from build123d import *

# Parameters (mm, degrees)
BOSS_EXTRUDE1_DEPTH = 165.1
SKETCH3_R           = 2.667
CUT_EXTRUDE1_DEPTH  = 165.1


with BuildPart() as part:
    # Sketch1 → Boss-Extrude1 (new body)
    with BuildSketch(Plane.XY):
        with BuildLine():
            Line((-5.08, 0), (5.08, 0))
            Line((5.08, 0), (5.08, 1.27))
            ThreePointArc((5.08, 1.27), (25.4, 15.895452724), (45.72, 1.27))
            Line((45.72, 1.27), (45.72, 0))
            Line((45.72, 0), (55.88, 0))
            Line((55.88, 0), (55.88, 3.161651537))
            Line((55.88, 3.161651537), (45.736301675, 3.161651537))
            ThreePointArc((45.736301675, 3.161651537), (25.4, 20.58060267), (5.063698325, 3.161651537))
            Line((5.063698325, 3.161651537), (-5.08, 3.161651537))
            Line((-5.08, 3.161651537), (-5.08, 0))
        make_face()
    extrude(amount=BOSS_EXTRUDE1_DEPTH)

    # Sketch3 → Cut-Extrude1 (cut)
    with BuildSketch(Plane(origin=(0, 3.161651537, 0), x_dir=(1, 0, 0), z_dir=(0, 1, 0))):
        with Locations(Location((0, -6.6675, 0), (0, 0, 270))):
            Circle(SKETCH3_R)
        with Locations(Location((0, -32.0675, 0), (0, 0, 270))):
            Circle(SKETCH3_R)
        with Locations(Location((0, -57.4675, 0), (0, 0, 270))):
            Circle(SKETCH3_R)
        with Locations(Location((0, -82.8675, 0), (0, 0, 270))):
            Circle(SKETCH3_R)
        with Locations(Location((0, -108.2675, 0), (0, 0, 270))):
            Circle(SKETCH3_R)
        with Locations(Location((0, -133.6675, 0), (0, 0, 270))):
            Circle(SKETCH3_R)
        with Locations(Location((0, -159.0675, 0), (0, 0, 270))):
            Circle(SKETCH3_R)
        with Locations(Location((50.8, -159.0675, 0), (0, 0, 180))):
            Circle(SKETCH3_R)
        with Locations(Location((50.8, -133.6675, 0), (0, 0, 180))):
            Circle(SKETCH3_R)
        with Locations(Location((50.8, -108.2675, 0), (0, 0, 180))):
            Circle(SKETCH3_R)
        with Locations(Location((50.8, -82.8675, 0), (0, 0, 180))):
            Circle(SKETCH3_R)
        with Locations(Location((50.8, -57.4675, 0), (0, 0, 180))):
            Circle(SKETCH3_R)
        with Locations(Location((50.8, -32.0675, 0), (0, 0, 180))):
            Circle(SKETCH3_R)
        with Locations(Location((50.8, -6.6675, 0), (0, 0, 180))):
            Circle(SKETCH3_R)
    extrude(amount=-CUT_EXTRUDE1_DEPTH, mode=Mode.SUBTRACT)


solid = part.part
Verification items for the finished model (mm, model axes). A direction names the side the tool comes from. Coordinates: 2 decimals unless noted, no trailing zeros. Loops run counter-clockwise (first coordinate to the right, second up) from the corner with the lowest first, then second, coordinate; pieces in that order, holes last. Notation, with made-up numbers: (29, -23.5) -> (79, -23.5) arc R28 cw to (79, -1.5) -> close; hole circle Ø1 at (83, 82). An arc over 180 degrees is marked (long way). Answer as a JSON object with one key per item and string values. Group by question number.
Item 1: Depth check by flat-ended pin: pin 1 (8.5 mm diameter, centred on x = 50.8, z = 82.87, fed in from -Y); pin 2 (1 mm diameter, centred on x = 36.5, z = 50.5, fed in from -Y); pin 3 (10 mm diameter, centred on x = 4.5, z = 33.5, fed in from +Y); pin 4 (6 mm diameter, centred on x = 0, z = 159.07, fed in from +Y). Enter the tip coordinate at first touch or a pass-through.
Item 2: Mould release check, pull along Z, two halves, no side actions. Record for faces 1 (the cylindrical face through (25.808, 20.577, 81.394)), 2 (the cylindrical face through (-1.02, 1.6, 59.93)), 3 (the flat face through (25.3, 16.4, 0)): +Z half, -Z half, draft (parallel to the pull), parting line (faces both ways), or undercut.
Item 3: Sectioned sample at B-B on y = 13.5. Record the boundary of the cut face in (x, z).
Item 4: Scan lines: probe 1 along X at (y, z) = (12.5, 99); probe 2 along Y at (x, z) = (49, 146); probe 3 along X at (y, z) = (5.75, 69). Record each from-to range of solid material in increasing order.
Item 5: Sectioned sample at C-C on z = 99. Record the boundary of the cut face in (x, y), plus the area to 3 significant figures.
Item 6: Tool access check on faces 4 (the cylindrical face through (-1.02, 1.6, 34.53)), 5 (the flat face through (3, 3.162, 81)), 6 (the flat face through (53, 3.162, 81)). Record the directions out of +Z, -Z, +X, -X, +Y, -Y that give a thin tool (end or side, any length) a straight path to the whole face; none if there is none.
Item 7: Sectioned sample at A-A on x = 50.8. State how many separate pieces and enclosed holes the cut face has, plus the area to 3 significant figures.
Item 8: Sectioned sample at D-D on x = 44. Record the boundary of the cut face in (y, z).
Evaluation:
{
 "1": {"pin 1": "stops at y = 0", "pin 2": "stops at y = 12.48", "pin 3": "stops at y = 13.07", "pin 4": "stops at y = 3.16"},
 "2": {"face 1": "draft", "face 2": "undercut", "face 3": "-Z half"},
 "3": {"outline": "(9.87, 0) -> (15.55, 0) -> (15.55, 165.1) -> (9.87, 165.1) -> close; (35.25, 0) -> (40.93, 0) -> (40.93, 165.1) -> (35.25, 165.1) -> close"},
 "4": {"probe 1": "x = 9.05 to 13.82, 36.98 to 41.75", "probe 2": "y = 0 to 3.16", "probe 3": "x = 5.64 to 7.18, 43.62 to 45.16"},
 "5": {"outline": "(-5.08, 0) -> (5.08, 0) -> (5.08, 1.27) arc R21.43 cw to (45.72, 1.27) -> (45.72, 0) -> (55.88, 0) -> (55.88, 3.16) -> (45.74, 3.16) arc R20.58 ccw to (5.06, 3.16) -> (-5.08, 3.16) -> close", "area": "242 mm²"},
 "6": {"face 4": "+Y, -Y", "face 5": "+Z, -Z, -X, +Y", "face 6": "+Z, -Z, +X, +Y"},
 "7": {"separate pieces": "8", "enclosed holes": "0", "area": "404 mm²"},
 "8": {"outline": "(5.11, 0) -> (8.81, 0) -> (8.81, 165.1) -> (5.11, 165.1) -> close"}
}
